Geometry: final body of the model. Coordinates: model frame, mm. Face numbers are marked on the shaded views. A direction names the side the tool comes from. Give positions to 0.01 mm unless a question says otherwise; leave off trailing zeros. Write each loop counter-clockwise with the first axis right and the second up, starting at its lowest first coordinate (ties: lowest second). Pieces come first, ordered by that corner, then holes. Notation, with made-up numbers: M -5.5,43 L 32.5,43 A28 ccw 32.5,76 Z; hole C -22,17 d7. An arc over 180 degrees is marked long. Use a Markdown table: item, result. Add a question column.
(1) Pin query (flat end, axial travel): pin 1 Ø5 at (y, z) = (-4, -1.5) entering from +X; pin 2 Ø5 at (y, z) = (-1, -4.5) entering from +X; pin 3 Ø2 at (y, z) = (-0.5, -8.5) entering from +X. Return the tip coordinate at first contact, or that it passes through.
(2) Cut plane C-C (x = 4.5). Output: boundary loops of the cut face in (y, z), plus the area to 3 significant figures.
(3) Cut plane D-D (z = -8). Output: boundary loops of the cut face in (x, y), plus the area to 3 significant figures.
(4) Material intervals for L1, parallel to Y at x = -14.5, z = -5.5; L2, parallel to X at y = -4.5, z = -7.75; L3, parallel to X at y = -7.5, z = -3.25, sorted ascending.
(5) Cut plane B-B (z = -5). Output: boundary loops of the cut face in (x, y).
(6) Cut plane A-A (y = 1.5). Output: boundary loops of the cut face in (x, z).
(7) Reachability of the marked faces 1, 2, 3 and 4 from +Z, -Z, +X, -X, +Y, -Y: full face, straight path, thin tool, end or side. Return the list, or none.
```python
from build123d import *

# Parameters (mm, degrees)
BOSS_EXTRUDE1_DEPTH = 10
BOSS_EXTRUDE2_DEPTH = 2


with BuildPart() as part:
    # Sketch1 → Boss-Extrude1 (new body, symmetric)
    with BuildSketch(Plane(origin=(0, 0, 0), x_dir=(1, 0, 0), z_dir=(0, 1, 0))):
        with BuildLine():
            Line((-25.066666667, 10.108740054), (-23.5, 11.351943801))
            ThreePointArc((-23.5, 11.351943801), (0, 0), (23.5, 11.351943801))
            Line((23.5, 11.351943801), (25.066666667, 10.108740054))
            ThreePointArc((25.066666667, 10.108740054), (0, -2), (-25.066666667, 10.108740054))
        make_face()
    extrude(amount=BOSS_EXTRUDE1_DEPTH, both=True)

    # Sketch2 → Boss-Extrude2 (add, symmetric)
    with BuildSketch(Plane(origin=(0, 0, 0), x_dir=(1, 0, 0), z_dir=(0, 1, 0))):
        with BuildLine():
            Line((-23.216373532, 11), (23.216373532, 11))
            ThreePointArc((23.216373532, 11), (0, 0), (-23.216373532, 11))
        make_face()
    extrude(amount=BOSS_EXTRUDE2_DEPTH, both=True)


solid = part.part
```
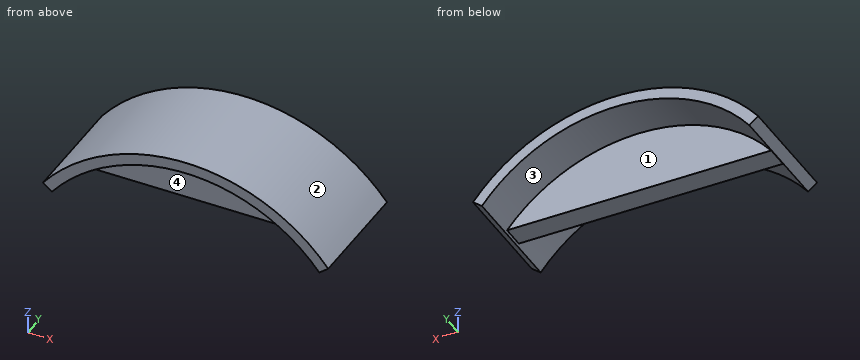
Answer list:
| question | item | result |
|---|---|---|
| 1 | pin 1 | x = 18.65 |
| 1 | pin 2 | x = 22.25 |
| 1 | pin 3 | x = 24.57 |
| 2 | outline | M -10,-0.34 L -2,-0.34 L -2,-11 L 2,-11 L 2,-0.34 L 10,-0.34 L 10,1.68 L -10,1.68 Z |
| 2 | area | 83.1 mm² |
| 3 | outline | M -23.24,-10 L -20.4,-10 L -20.4,-2 L 20.4,-2 L 20.4,-10 L 23.24,-10 L 23.24,10 L 20.4,10 L 20.4,2 L -20.4,2 L -20.4,10 L -23.24,10 Z |
| 3 | area | 277 mm² |
| 4 | L1 | -2 to 2 |
| 4 | L2 | -23 to -20.12, 20.12 to 23 |
| 4 | L3 | -17.56 to -13.58, 13.58 to 17.56 |
| 5 | outline | M -19.97,-10 L -16.58,-10 L -16.58,-2 L 16.58,-2 L 16.58,-10 L 19.97,-10 L 19.97,10 L 16.58,10 L 16.58,2 L -16.58,2 L -16.58,10 L -19.97,10 Z |
| 6 | outline | M -25.07,-10.11 L -23.5,-11.35 A30 cw -23.22,-11 L 23.22,-11 A30 cw 23.5,-11.35 L 25.07,-10.11 A32 ccw Z |
| 7 | face 1 | -Z, +Y |
| 7 | face 2 | +Z, +Y, -Y |
| 7 | face 3 | -Z |
| 7 | face 4 | -Z, -Y |
